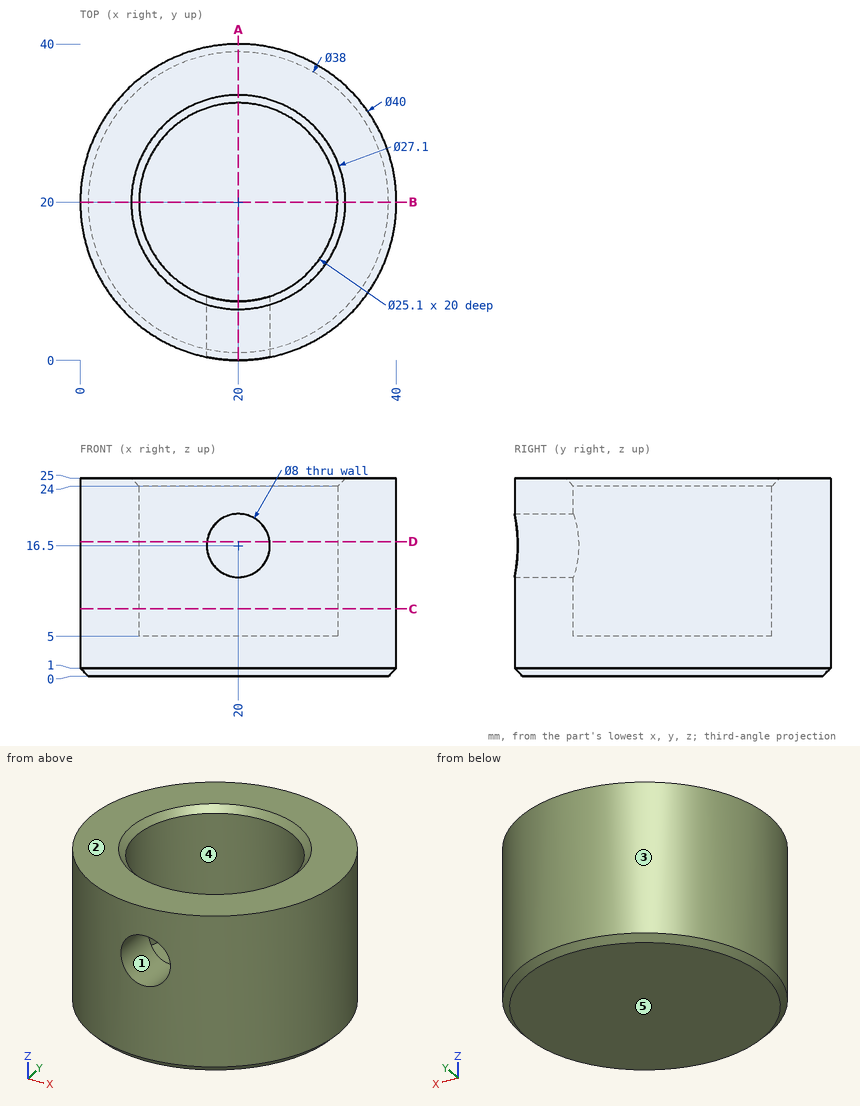
Could you check a few things on this drawing? It's one solid part, dimensions in mm from its lowest x, y, z. A direction names the side the tool comes from. Give positions to 0.01 mm unless a question says otherwise; leave off trailing zeros. Loops run counter-clockwise (first coordinate to the right, second up) from the corner with the lowest first, then second, coordinate; pieces in that order, holes last. Notation, with made-up numbers: (-19, -22.5) -> (-9, -22.5) arc R25 cw to (-9, 8.5) -> close; hole circle Ø2 at (14.25, 63). An arc over 180 degrees is marked (long way). Answer as CSV lines item,"result". Start each with the question number.
(1) If we section it at B-B on y = 20: Write out the boundary of the cut face in (x, z).
(2) We'd pull the mould along X, two halves only. Please class the marked faces 3, 4 and 5: released by +X, released by -X, zero draft, split by the parting line, or undercut.
(3) Which directions (+Z, -Z, +X, -X, +Y, -Y) give clear straight access to the entire face, cutting with the end or side of a thin tool? Please do the marked faces 1 and 2.
(4) I'm going to push flat-ended pins straight in: pin 1 Ø5 at (x, y) = (9, 27) entering from +Z; pin 2 Ø6 at (x, z) = (26, 10) entering from +Y; pin 3 Ø12 at (x, z) = (35.5, 7) entering from +Y; pin 4 Ø3 at (x, z) = (28.5, 15.5) entering from +Y (3 decimals). Where does each tip first touch, or does it pass through?
(5) If we section it at C-C on z = 8.5: Write out the boundary of the cut face in (x, y), then the cut area to 3 significant figures.
(6) If we section it at A-A on x = 20: Write out the boundary of the cut face in (y, z).
(7) If we section it at D-D on z = 17: Write out the boundary of the cut face in (x, y), then the cut area to 3 significant figures.
(8) I need wall thicknesses on probe 1 along Z at (x, y) = (20, 6); probe 2 along X at (y, z) = (19.5, 16.25); probe 3 along Y at (x, z) = (12, 15). Which ranges of each line are inside material? Lowest first, please.
Computed:
1,outline,"(0, 1) -> (1, 0) -> (39, 0) -> (40, 1) -> (40, 25) -> (33.55, 25) -> (32.55, 24) -> (32.55, 5) -> (7.45, 5) -> (7.45, 24) -> (6.45, 25) -> (0, 25) -> close"
2,face 3,"split by the parting line"
2,face 4,"undercut"
2,face 5,"zero draft"
3,face 1,"-Y"
3,face 2,"+Z, +X, -X, +Y, -Y"
4,pin 1,"stops at z = 25"
4,pin 2,"stops at y = 39.77"
4,pin 3,"stops at y = 37.6"
4,pin 4,"stops at y = 38.735"
5,outline,"circle Ø40 at (20, 20); hole circle Ø25.1 at (20, 20)"
5,area,"762 mm2"
6,outline,"(0, 1) -> (1, 0) -> (39, 0) -> (40, 1) -> (40, 25) -> (33.55, 25) -> (32.55, 24) -> (32.55, 5) -> (7.45, 5) -> (7.45, 12.5) -> (0, 12.5) -> close; (0, 20.5) -> (7.45, 20.5) -> (7.45, 24) -> (6.45, 25) -> (0, 25) -> close"
7,outline,"(16.03, 0.4) -> (16.03, 8.09) arc R12.55 cw (long way) to (23.97, 8.09) -> (23.97, 0.4) arc R20 ccw (long way) to start"
7,area,"702 mm2"
8,probe 1,"z = 0 to 12.5, 20.5 to 25"
8,probe 2,"x = 0.01 to 7.46, 32.54 to 39.99"
8,probe 3,"y = 1.67 to 10.33, 29.67 to 38.33"
